Part model, mm, in its own coordinate system. Face numbers are marked on the shaded views. A direction names the side the tool comes from. Round coordinates to 2 decimals unless told otherwise and drop trailing zeros. Order: outer loops, then holes, each group sorted by start corner. A loop starts at its lowest first (then second) coordinate and runs counter-clockwise, first axis right, second up. Notation, with made-up numbers: (67.25, 51.25) - (102.25, 51.25) arc R19 ccw to (102.25, 73.25) - close; hole circle Ø6 at (-9.5, -19.5). An arc over 180 degrees is marked (long way). Return JSON: item names as keys, results as strings. Group by question number.
Item 1: Saw through at D-D on y = -11. List the corners of the cut face in (x, z).
Item 2: Saw through at A-A on x = 10. List the corners of the cut face in (y, z), and give its area (3 significant figures).
Item 3: Tool access for the marked faces 1 and 2: list every direction of +Z, -Z, +X, -X, +Y, -Y with a clear straight run to the whole face (end or side of a thin tool).
Item 4: Drop flat-ended pins along their axis: pin 1 (5 mm diameter, centred on y = -22, z = 11.5, fed in from -X); pin 2 (5 mm diameter, centred on x = 10, z = -11, fed in from -Y). Give the stop position or say it passes through.
Item 5: Saw through at B-B on y = -2.5. List the corners of the cut face in (x, z).
Item 6: Saw through at C-C on z = 11. List the corners of the cut face in (x, y), and give its area (3 significant figures).
Item 7: Probe probe 1 along X at (y, z) = (1.35, 11); probe 2 along Y at (x, z) = (25, 0); probe 3 along X at (y, z) = (1.5, -10). List the from-to ranges inside material, lowest first.
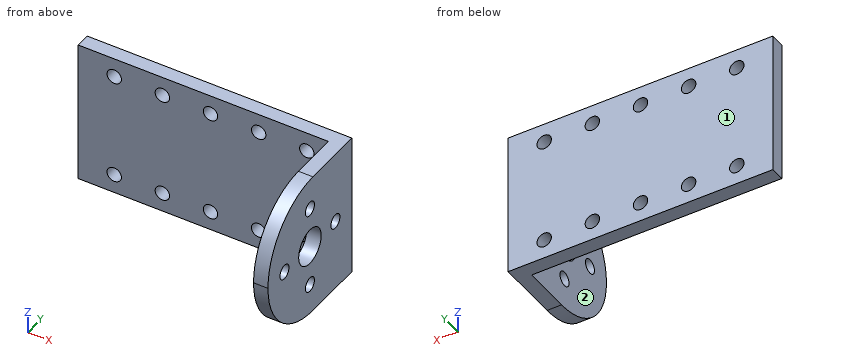
```python
from build123d import *

# Parameters (mm, degrees)
SKETCH1_W           = 55
SKETCH1_H           = 30
SKETCH1_R           = 1.5
BOSS_EXTRUDE1_DEPTH = 3
SKETCH2_W           = 3
SKETCH2_H           = 30
BOSS_EXTRUDE2_DEPTH = 25
SKETCH3_R           = 1.5
SKETCH3_R_2         = 3.75
CUT_EXTRUDE1_DEPTH  = 3
FILLET1_R           = 15


with BuildPart() as part:
    # Sketch1 → Boss-Extrude1 (new body)
    with BuildSketch(Plane(origin=(0, 0, 0), x_dir=(1, 0, 0), z_dir=(0, 1, 0))):
        Rectangle(SKETCH1_W, SKETCH1_H)
        with Locations(Location((20, 11, 0), (0, 0, 270))):
            Circle(SKETCH1_R, mode=Mode.SUBTRACT)
        with Locations(Location((10, 11, 0), (0, 0, 270))):
            Circle(SKETCH1_R, mode=Mode.SUBTRACT)
        with Locations(Location((0, 11, 0), (0, 0, 270))):
            Circle(SKETCH1_R, mode=Mode.SUBTRACT)
        with Locations(Location((-10, 11, 0), (0, 0, 270))):
            Circle(SKETCH1_R, mode=Mode.SUBTRACT)
        with Locations(Location((-20, 11, 0), (0, 0, 270))):
            Circle(SKETCH1_R, mode=Mode.SUBTRACT)
        with Locations(Location((20, -11, 0), (0, 0, 90))):
            Circle(SKETCH1_R, mode=Mode.SUBTRACT)
        with Locations(Location((10, -11, 0), (0, 0, 90))):
            Circle(SKETCH1_R, mode=Mode.SUBTRACT)
        with Locations(Location((0, -11, 0), (0, 0, 90))):
            Circle(SKETCH1_R, mode=Mode.SUBTRACT)
        with Locations(Location((-10, -11, 0), (0, 0, 90))):
            Circle(SKETCH1_R, mode=Mode.SUBTRACT)
        with Locations(Location((-20, -11, 0), (0, 0, 90))):
            Circle(SKETCH1_R, mode=Mode.SUBTRACT)
    extrude(amount=BOSS_EXTRUDE1_DEPTH)

    # Sketch2 → Boss-Extrude2 (add)
    with BuildSketch(Plane.XZ):
        with Locations((26, 0)):
            Rectangle(SKETCH2_W, SKETCH2_H)
    extrude(amount=BOSS_EXTRUDE2_DEPTH)

    # Sketch3 → Cut-Extrude1 (cut)
    with BuildSketch(Plane(origin=(27.5, 0, 0), x_dir=(0, 0, -1), z_dir=(1, 0, 0))):
        with Locations((0, -19.5)):
            Circle(SKETCH3_R)
        with Locations((-8.5, -11)):
            Circle(SKETCH3_R)
        with Locations((0, -2.5)):
            Circle(SKETCH3_R)
        with Locations((8.5, -11)):
            Circle(SKETCH3_R)
        with Locations((0, -11)):
            Circle(SKETCH3_R_2)
    extrude(amount=-CUT_EXTRUDE1_DEPTH, mode=Mode.SUBTRACT)

    # Fillet1
    fillet1_edges = [part.edges().sort_by_distance(p)[0] for p in [
        (26, -25, -15),
        (26, -25, 15),
    ]]
    fillet(fillet1_edges, radius=FILLET1_R - 0.0001)  # a hair under: the kernel refuses the full size


solid = part.part
```
Filled in:
{
 "1": {"outline": "(24.5, -14.97) - (27.5, -14.97) - (27.5, -10) - (24.5, -10) - close; (24.5, -7) - (27.5, -7) - (27.5, -3.75) - (24.5, -3.75) - close; (24.5, 3.75) - (27.5, 3.75) - (27.5, 7) - (24.5, 7) - close; (24.5, 10) - (27.5, 10) - (27.5, 14.97) - (24.5, 14.97) - close"},
 "2": {"outline": "(0, -15) - (3, -15) - (3, -12.5) - (0, -12.5) - close; (0, -9.5) - (3, -9.5) - (3, 9.5) - (0, 9.5) - close; (0, 12.5) - (3, 12.5) - (3, 15) - (0, 15) - close", "area": "72.0 mm^2"},
 "3": {"face 1": "+Z, -Z, +X, -X, +Y", "face 2": "+Z, -Z, -X, -Y"},
 "4": {"pin 1": "stops at x = 24.5", "pin 2": "stops at y = 0"},
 "5": {"outline": "(24.5, -15) - (27.5, -15) - (27.5, -1.5) - (24.5, -1.5) - close; (24.5, 1.5) - (27.5, 1.5) - (27.5, 15) - (24.5, 15) - close"},
 "6": {"outline": "(-27.5, 0) - (-21.5, 0) - (-21.5, 3) - (-27.5, 3) - close; (-18.5, 0) - (-11.5, 0) - (-11.5, 3) - (-18.5, 3) - close; (-8.5, 0) - (-1.5, 0) - (-1.5, 3) - (-8.5, 3) - close; (1.5, 0) - (8.5, 0) - (8.5, 3) - (1.5, 3) - close; (11.5, 0) - (18.5, 0) - (18.5, 3) - (11.5, 3) - close; (21.5, 0) - (24.5, 0) - (24.5, -20.2) - (27.5, -20.2) - (27.5, 3) - (21.5, 3) - close", "area": "181 mm^2"},
 "7": {"probe 1": "x = -27.5 to -21.5, -18.5 to -11.5, -8.5 to -1.5, 1.5 to 8.5, 11.5 to 18.5, 21.5 to 27.5", "probe 2": "y = -25 to -21, -18 to -14.75, -7.25 to -4, -1 to 3", "probe 3": "x = -27.5 to -21.12, -18.88 to -11.12, -8.88 to -1.12, 1.12 to 8.88, 11.12 to 18.88, 21.12 to 27.5"}
}
